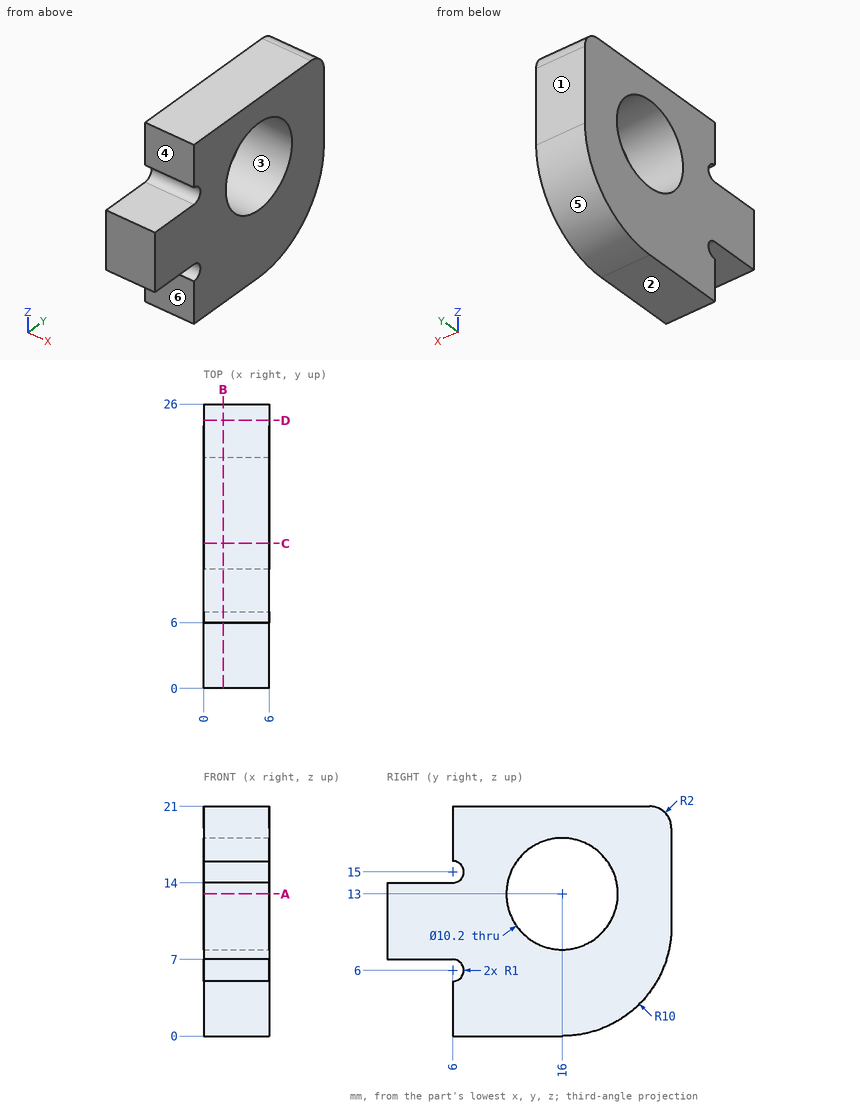
Study the drawing (mm; zero at the part's minimum x, y, z) and answer. A direction names the side the tool comes from. Give positions to 0.01 mm unless a question says otherwise; leave off trailing zeros. Loops run counter-clockwise (first coordinate to the right, second up) from the corner with the lowest first, then second, coordinate; pieces in that order, holes last. Notation, with made-up numbers: M 77.25,-19.75 L 95.25,-19.75 A18 cw 95.25,5.25 Z; hole C 22.25,70.5 d3. An arc over 180 degrees is marked long. One line per item, written item: value.
1. Section C-C on y = 13.25 is taken. Determine the outline of the cut face in (x, z).
Found:
outline: M 0,0 L 6,0 L 6,8.7 L 0,8.7 Z; M 0,17.3 L 6,17.3 L 6,21 L 0,21 Z
2. For a pull along Z with two mould halves and no side action, classify the marked faces 1, 2 and 3 as pulls with the +Z half, pulls with the -Z half, needs draft (parallel to the pull), parting line crosses it, or undercut.
Found:
face 1: needs draft
face 2: pulls with the -Z half
face 3: undercut
3. Section B-B on x = 1.8 is taken. Determine the outline of the cut face in (y, z).
Found:
outline: M 0,7 L 6,7 A1 cw 6,5 L 6,0 L 16,0 A10 ccw 26,10 L 26,19 A2 ccw 24,21 L 6,21 L 6,16 A1 cw 6,14 L 0,14 Z; hole C 16,13 d10.2
4. Find the intervals of material crossed by probe 1 along Y at (x, z) = (3.7, 13); probe 2 along Z at (x, y) = (4.35, 2); probe 3 along Y at (x, z) = (5.6, 11), in increasing order.
Found:
probe 1: 0 to 10.9, 21.1 to 26
probe 2: 7 to 14
probe 3: 0 to 11.31, 20.69 to 26
5. Section A-A on z = 13 is taken. Determine the outline of the cut face in (x, y), plus the area to 3 significant figures.
Found:
outline: M 0,0 L 6,0 L 6,10.9 L 0,10.9 Z; M 0,21.1 L 6,21.1 L 6,26 L 0,26 Z
area: 94.8 mm^2
6. Each of these flat-tipped pins is pushed along its axis until it touches: P1, Ø11.5, axis at y = 16, z = 13, coming from the +X side; P2, Ø3, axis at x = 1, z = 3.5, coming from the +Y side; P3, Ø3, axis at x = 4.5, y = 3.5, coming from the -Z side. Where does it stop, or does it pass through?
Found:
P1: x = 6
P2: y = 24.66
P3: z = 7
7. For the marked faces 4, 5 and 6, determine the directions among +Z, -Z, +X, -X, +Y, -Y from which every point of the face is accessible in a straight line to the end or side of a thin tool.
Found:
face 4: +Z, +X, -X, -Y
face 5: -Z, +X, -X, +Y
face 6: -Z, +X, -X, -Y
8. Section D-D on y = 24.5 is taken. Determine the outline of the cut face in (x, z).
Found:
outline: M 0,4.73 L 6,4.73 L 6,20.94 L 0,20.94 Z
